from build123d import *

# Parameters (mm, degrees)
SKETCH_1_W          = 60
SKETCH_1_H          = 80
EXTRUDE_1_DEPTH     = 45
SKETCH_2_R          = 1.35
CUT_EXTRUDE_1_DEPTH = 100
SKETCH_3_R          = 1.65
CUT_EXTRUDE_2_DEPTH = 100
SKETCH_4_R          = 5.25
CUT_EXTRUDE_3_DEPTH = 1000
SKETCH_5_W          = 48
SKETCH_5_H          = 33
CUT_EXTRUDE_4_DEPTH = 25
SKETCH_6_R          = 1.65
CUT_EXTRUDE_5_DEPTH = 5000


with BuildPart() as part:
    # 草图1 → 凸台-拉伸1 (new body)
    with BuildSketch(Plane.XY):
        Rectangle(SKETCH_1_W, SKETCH_1_H)
    extrude(amount=EXTRUDE_1_DEPTH)

    # 草图2 → 切除-拉伸1 (cut)
    with BuildSketch(Plane.XY.offset(45)):
        with Locations((17.5, -30)):
            Circle(SKETCH_2_R)
        with Locations((-17.5, -30)):
            Circle(SKETCH_2_R)
    extrude(amount=-CUT_EXTRUDE_1_DEPTH, mode=Mode.SUBTRACT)

    # 草图3 → 切除-拉伸2 (cut)
    with BuildSketch(Plane.XY.offset(45)):
        with Locations((8, 4)):
            Circle(SKETCH_3_R)
        with Locations((0, 12)):
            Circle(SKETCH_3_R)
        with Locations((-8, 4)):
            Circle(SKETCH_3_R)
        with Locations((0, -4)):
            Circle(SKETCH_3_R)
    extrude(amount=-CUT_EXTRUDE_2_DEPTH, mode=Mode.SUBTRACT)

    # 草图4 → 切除-拉伸3 (cut)
    with BuildSketch(Plane.XY.offset(45)):
        with Locations((0, 4)):
            Circle(SKETCH_4_R)
    extrude(amount=-CUT_EXTRUDE_3_DEPTH, mode=Mode.SUBTRACT)

    # 草图5 → 切除-拉伸4 (cut)
    with BuildSketch(Plane.XZ.offset(40)):
        with Locations((0, 22.5)):
            Rectangle(SKETCH_5_W, SKETCH_5_H)
    extrude(amount=-CUT_EXTRUDE_4_DEPTH, mode=Mode.SUBTRACT)

    # 草图6 → 切除-拉伸5 (cut)
    with BuildSketch(Plane(origin=(30, 0, 0), x_dir=(0, 0, -1), z_dir=(1, 0, 0))):
        with Locations((-18, 30)):
            Circle(SKETCH_6_R)
        with Locations((-27, 30)):
            Circle(SKETCH_6_R)
    extrude(amount=-CUT_EXTRUDE_5_DEPTH, mode=Mode.SUBTRACT)


solid = part.part
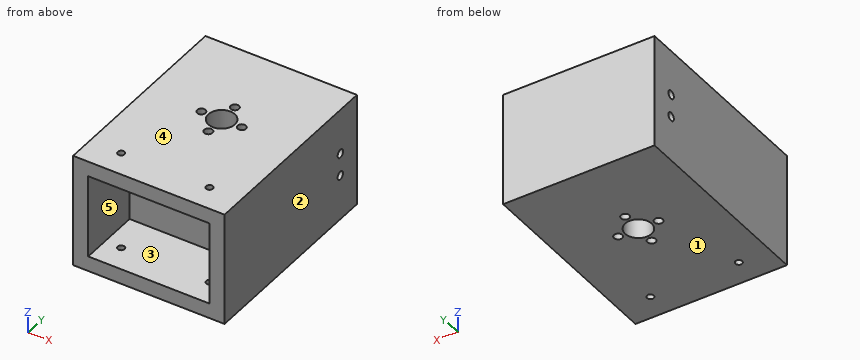
Check sheet for the modelled part. Datum: model origin and axes. Units: mm. Face numbers are marked on the shaded views. A direction names the side the tool comes from. Round coordinates to 2 decimals unless told otherwise and drop trailing zeros. Loops run counter-clockwise (first coordinate to the right, second up) from the corner with the lowest first, then second, coordinate; pieces in that order, holes last.
1. Mould release check, pull along Z, two halves, no side actions. Record for the marked faces 1, 2 and 3: released by +Z, released by -Z, zero draft, split by the parting line, or undercut.
2. Set-up check for the marked faces 4 and 5: record each of +Z, -Z, +X, -X, +Y, -Y from which the full face is reachable in a straight line by a thin tool's end or side.
3. Gauge pin test, flat end, axial feed: pin 1 Ø8 at (x, z) = (-17, 16.5) entering from -Y. Record the tip position at first contact, or that the pin passes through.
4. Sectioned sample at A-A on z = 18. Record the boundary of the cut face in (x, y).
5. Sectioned sample at B-B on x = -8. Record the boundary of the cut face in (y, z), and give its area (3 significant figures).
6. Sectioned sample at C-C on y = 4. Record the boundary of the cut face in (x, z), and give its area (3 significant figures).
7. Sectioned sample at D-D on y = 12. Record the boundary of the cut face in (x, z).
8. Scan lines: probe 1 along Y at (x, z) = (0, 36); probe 2 along Z at (x, y) = (7, -28); probe 3 along Y at (x, z) = (17.5, 4.1). Record each from-to range of solid material in increasing order.
Recorded:
1. face 1: released by -Z
1. face 2: zero draft
1. face 3: undercut
2. face 4: +Z, +X, -X, +Y, -Y
2. face 5: -Y
3. pin 1: stops at y = -15
4. outline: (-30, -40) - (-24, -40) - (-24, -15) - (24, -15) - (24, -40) - (30, -40) - (30, 28.35) - (-30, 28.35) - close; (-30, 31.65) - (30, 31.65) - (30, 40) - (-30, 40) - close; hole circle Ø3.3 at (-8, 4); hole circle Ø10.5 at (0, 4); hole circle Ø3.3 at (0, -4); hole circle Ø3.3 at (0, 12); hole circle Ø3.3 at (8, 4)
5. outline: (-40, 0) - (2.35, 0) - (2.35, 45) - (-40, 45) - (-40, 39) - (-15, 39) - (-15, 6) - (-40, 6) - close; (5.65, 0) - (40, 0) - (40, 45) - (5.65, 45) - close; hole circle Ø3.3 at (30, 18); hole circle Ø3.3 at (30, 27)
5. area: 2,610 mm2
6. outline: (-30, 0) - (-9.65, 0) - (-9.65, 45) - (-30, 45) - close; (-6.35, 0) - (-5.25, 0) - (-5.25, 45) - (-6.35, 45) - close; (5.25, 0) - (6.35, 0) - (6.35, 45) - (5.25, 45) - close; (9.65, 0) - (30, 0) - (30, 45) - (9.65, 45) - close
6. area: 1,930 mm2
7. outline: (-30, 0) - (-1.65, 0) - (-1.65, 45) - (-30, 45) - close; (1.65, 0) - (30, 0) - (30, 45) - (1.65, 45) - close
8. probe 1: y = -15 to -5.65, -2.35 to -1.25, 9.25 to 10.35, 13.65 to 40
8. probe 2: z = 0 to 6, 39 to 45
8. probe 3: y = -40 to -31.35, -28.65 to 40
